from build123d import *

# Parameters (mm, degrees)
SKETCH1_W           = 100
SKETCH1_H           = 50
BOSS_EXTRUDE1_DEPTH = 5
CUT_EXTRUDE1_DEPTH  = 10
CUT_EXTRUDE2_DEPTH  = 57.124860802
EXTRUDE_THIN2_START = -5
EXTRUDE_THIN2_DEPTH = 5
BOSS_EXTRUDE3_DEPTH = 5
SKETCH7_R           = 6.5
CUT_EXTRUDE3_DEPTH  = 57.124860802
SKETCH8_R           = 0.5
CUT_EXTRUDE4_DEPTH  = 57.124860802


# Read off the part's stored shape, not the designer's step: Extrude-Thin2
with BuildPart() as part:
    # Sketch1 → Boss-Extrude1 (new body)
    with BuildSketch(Plane(origin=(0, 0, 0), x_dir=(1, 0, 0), z_dir=(0, 1, 0))):
        Rectangle(SKETCH1_W, SKETCH1_H)
    extrude(amount=BOSS_EXTRUDE1_DEPTH)

    # Sketch2 → Cut-Extrude1 (cut)
    with BuildSketch(Plane(origin=(0, 5, 0), x_dir=(1, 0, 0), z_dir=(0, 1, 0))):
        Polygon((23.5, -11.258330249), (36.5, -11.258330249), (43, 0), (36.5, 11.258330249), (23.5, 11.258330249), (17, 0), align=None)
    extrude(amount=-CUT_EXTRUDE1_DEPTH, mode=Mode.SUBTRACT)

    # Sketch3 → Cut-Extrude2 (cut, through all)
    with BuildSketch(Plane(origin=(0, 5, 0), x_dir=(1, 0, 0), z_dir=(0, 1, 0))):
        Polygon((50, -25), (-50, -10), (-50, -25), align=None)
    cut_extrude2 = extrude(amount=-CUT_EXTRUDE2_DEPTH, mode=Mode.SUBTRACT)

    # Mirror1: Cut-Extrude2 across plane
    add(cut_extrude2.mirror(Plane.XY), mode=Mode.SUBTRACT)

    # Extrude-Thin2 outline → Extrude-Thin2 (add)
    with BuildSketch(Plane(origin=(0, 5, 0), x_dir=(1, 0, 0), z_dir=(0, 1, 0)).offset(EXTRUDE_THIN2_START)):
        Polygon((17, 0), (17.288675135, -0.5), (29.711324865, -0.5), (35.922649731, -11.258330249), (36.5, -11.258330249), (36.788675135, -10.758330249), (30.577350269, 0), (36.788675135, 10.758330249), (36.5, 11.258330249), (35.922649731, 11.258330249), (29.711324865, 0.5), (17.288675135, 0.5), align=None)
    extrude(amount=EXTRUDE_THIN2_DEPTH)

    # Sketch6 → Boss-Extrude3 (add, through all)
    with BuildSketch(Plane(origin=(0, 5, 0), x_dir=(1, 0, 0), z_dir=(0, 1, 0))):
        Polygon((31.5, 0), (30.75, 1.299038106), (29.25, 1.299038106), (28.5, 0), (29.25, -1.299038106), (30.75, -1.299038106), align=None)
    extrude(amount=-BOSS_EXTRUDE3_DEPTH)

    # Sketch7 → Cut-Extrude3 (cut, through all)
    with BuildSketch(Plane(origin=(0, 5, 0), x_dir=(1, 0, 0), z_dir=(0, 1, 0))):
        with Locations(Location((-40, 0, 0), (0, 0, 270))):
            Circle(SKETCH7_R)
    extrude(amount=-CUT_EXTRUDE3_DEPTH, mode=Mode.SUBTRACT)

    # Sketch8 → Cut-Extrude4 (cut, through all)
    with BuildSketch(Plane(origin=(0, 5, 0), x_dir=(1, 0, 0), z_dir=(0, 1, 0))):
        with Locations(Location((30, 0, 0), (0, 0, 270))):
            Circle(SKETCH8_R)
    extrude(amount=-CUT_EXTRUDE4_DEPTH, mode=Mode.SUBTRACT)


solid = part.part
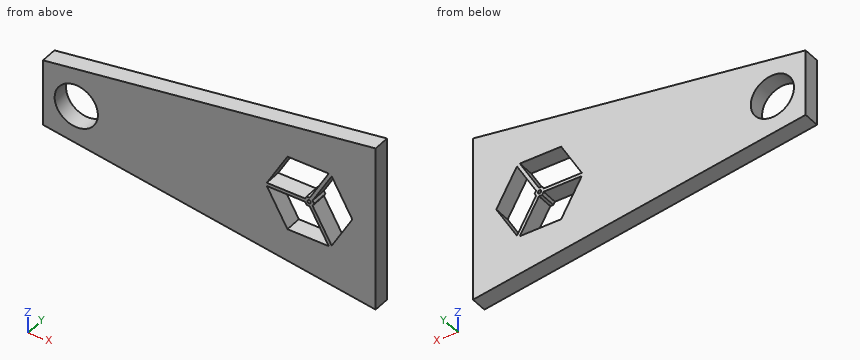
Could you check a few things on this model? Use its own coordinates, in mm. Give positions to 0.01 mm unless a question says otherwise; leave off trailing zeros. Order: outer loops, then holes, each group sorted by start corner. A loop starts at its lowest first (then second) coordinate and runs counter-clockwise, first axis right, second up.
1. Suppose I cut it at C-C (z = -5). List the corners of the cut face in (x, y) for me.
2. Suppose I cut it at A-A (x = -40). List the corners of the cut face in (y, z) for me.
3. Suppose I cut it at B-B (y = 0.95). List the corners of the cut face in (x, z) for me.
4. I need wall thicknesses on L1, parallel to X at y = 3.8, z = -5; L2, parallel to X at y = 2.35, z = 9; L3, parallel to Z at x = 26, y = 0.5. Which ranges of each line are inside material? Lowest first, please.
5. Suppose I cut it at D-D (x = -3). List the corners of the cut face in (y, z) for me.
6. Will these pins go through, and if not, where does the flat tip stop? P1, Ø2.5, axis at x = 31.5, y = 3.5, coming from the -Z side; P2, Ø4, axis at x = 24.5, z = -6, coming from the -Y side; P3, Ø1, axis at x = 29.5, y = 2.5, coming from the +Z side.
Solved:
1. outline: (-50, 0) - (-44.15, 0) - (-44.15, 5) - (-50, 5) - close; (-35.85, 0) - (19.89, 0) - (19.89, 5) - (-35.85, 5) - close; (32.31, 0) - (33.46, 0) - (33.46, 5) - (32.31, 5) - close; (40.11, 0) - (50, 0) - (50, 5) - (40.11, 5) - close
2. outline: (0, -11.5) - (5, -11.5) - (5, -6.5) - (0, -6.5) - close; (0, 6.5) - (5, 6.5) - (5, 11.5) - (0, 11.5) - close
3. outline: (-50, -10) - (50, -25) - (50, 25) - (-50, 10) - close; hole circle Ø13 at (-40, 0); hole (17.29, -0.5) - (23.5, -11.26) - (35.92, -11.26) - (30.17, -1.3) - (29.25, -1.3) - (28.79, -0.5) - close; hole (17.29, 0.5) - (28.79, 0.5) - (29.25, 1.3) - (30.17, 1.3) - (35.92, 11.26) - (23.5, 11.26) - close; hole circle Ø1 at (30, 0); hole (31.04, -0.8) - (36.79, -10.76) - (43, 0) - (36.79, 10.76) - (31.04, 0.8) - (31.5, 0) - close
4. L1: x = -50 to -44.15, -35.85 to 19.89, 32.31 to 33.46, 40.11 to 50
4. L2: x = -50 to 22.2, 34.62 to 35.77, 37.8 to 50
4. L3: z = -21.4 to -11.26, -0.5 to 0.5, 11.26 to 21.4
5. outline: (0, -17.05) - (5, -17.05) - (5, 17.05) - (0, 17.05) - close
6. P1: stops at z = -22.41
6. P2: passes through
6. P3: stops at z = 22
